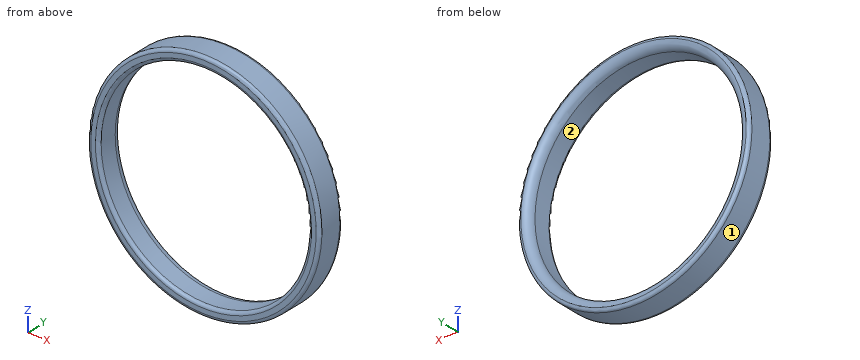
```python
from build123d import *

# Parameters (mm, degrees)
SKETCH1_R           = 7.4
SKETCH1_R_2         = 6.7
BOSS_EXTRUDE1_DEPTH = 1.8
FILLET1_R           = 0.5
FILLET2_R           = 0.2


with BuildPart() as part:
    # Sketch1 → Boss-Extrude1 (new body)
    with BuildSketch(Plane(origin=(0, 0, 0), x_dir=(1, 0, 0), z_dir=(0, 1, 0))):
        with Locations(Location((0, 0, 0), (0, 0, 270))):
            Circle(SKETCH1_R)
        with Locations(Location((0, 0, 0), (0, 0, 270))):
            Circle(SKETCH1_R_2, mode=Mode.SUBTRACT)
    extrude(amount=BOSS_EXTRUDE1_DEPTH)

    # Fillet1
    fillet1_edges = [part.edges().sort_by_distance(p)[0] for p in [
        (0, 1.8, -6.7),
    ]]
    fillet(fillet1_edges, radius=FILLET1_R)

    # Fillet2
    fillet2_edges = [part.edges().sort_by_distance(p)[0] for p in [
        (0, 0, -7.4),
        (0, 1.8, -7.4),
        (0, 0, -6.7),
    ]]
    fillet(fillet2_edges, radius=FILLET2_R - 0.0001)  # a hair under: the kernel refuses the full size


solid = part.part
```
Input: part model. Units: mm. Frame: model coordinates. Face numbers are marked on the shaded views. Coordinates: 2 decimals unless noted, no trailing zeros. Loops run counter-clockwise (first coordinate to the right, second up) from the corner with the lowest first, then second, coordinate; pieces in that order, holes last. Notation, with made-up numbers: M -12,6.5 L 27,6.5 A24 ccw 27,38.5 Z; hole C 14.5,46 d8. An arc over 180 degrees is marked long. Answer in a Markdown table with one row per item.
1. First-contact query: pin 1 (6 mm diameter, centred on x = -2, z = 5, fed in from +Y). Flat tip, straight axial feed; report the tip coordinate or a pass-through.
Response:
| item | result |
|---|---|
| pin 1 | stops at y = 1.8 |
2. Draft query along X for the marked faces 1 and 2. Return one class per face: pulls with the +X half, pulls with the -X half, needs draft (parallel to the pull), parting line crosses it, or undercut.
Response:
| item | result |
|---|---|
| face 1 | parting line crosses it |
| face 2 | undercut |
3. Material intervals for line 1 (X direction, y = 0.55, z = 0); line 2 (Z direction, x = 4, y = 0.4); line 3 (X direction, y = 0.3, z = 1.5), sorted ascending.
Response:
| item | result |
|---|---|
| line 1 | x = -7.4 to -6.7, 6.7 to 7.4 |
| line 2 | z = -6.23 to -5.37, 5.37 to 6.23 |
| line 3 | x = -7.25 to -6.53, 6.53 to 7.25 |
4. Section C-C, the plane y = 0.55. Output: boundary loops of the cut face in (x, z).
Response:
| item | result |
|---|---|
| outline | C 0,0 d14.8; hole C 0,0 d13.4 |
